Autodesk Fusion 360 part; units mm, degrees
sketch "Sketch1" plane through (0, 0, 0) normal (0, 0, 1) x (1, 0, 0)
  line L0 (-4.25, 7.25) -> (4.25, 7.25)
  line L1 (7.25, 4.25) -> (7.25, -4.25)
  line L2 (4.25, -7.25) -> (-4.25, -7.25)
  line L3 (-7.25, -4.25) -> (-7.25, 4.25)
  line L4 (-7.25, 7.25) -> (7.25, -7.25) construction
  line L5 (7.25, 7.25) -> (-7.25, -7.25) construction
  arc A0 (-4.25, 7.25) -> (-7.25, 4.25) centre (-4.25, 4.25) ccw
  arc A1 (-7.25, -4.25) -> (-4.25, -7.25) centre (-4.25, -4.25) ccw
  arc A2 (4.25, -7.25) -> (7.25, -4.25) centre (4.25, -4.25) ccw
  arc A3 (7.25, 4.25) -> (4.25, 7.25) centre (4.25, 4.25) ccw
  line L6 (10, 10) -> (-10, 10)
  line L7 (-15, 5) -> (-15, -5)
  line L8 (-10, -10) -> (10, -10)
  line L9 (15, -5) -> (15, 5)
  line L10 (15, 10) -> (-15, -10) construction
  line L11 (-15, 10) -> (15, -10) construction
  arc A4 (15, 5) -> (10, 10) centre (10, 5) ccw
  arc A5 (-10, 10) -> (-15, 5) centre (-10, 5) ccw
  arc A6 (-15, -5) -> (-10, -10) centre (-10, -5) ccw
  arc A7 (10, -10) -> (15, -5) centre (10, -5) ccw
  circle A8 centre (-12.5, 0) radius 1.6
  line L12 (0, 0) -> (0, 5.6259) construction
  circle A9 centre (12.5, 0) radius 1.6
  line L13 (-5.5, 2.65) -> (5.5, 2.65)
  line L14 (5.5, 2.65) -> (5.5, -2.65)
  line L15 (5.5, -2.65) -> (-5.5, -2.65)
  line L16 (-5.5, -2.65) -> (-5.5, 2.65)
  line L17 (-5.5, 2.65) -> (5.5, -2.65) construction
  line L18 (5.5, 2.65) -> (-5.5, -2.65) construction
  line L19 (-5.5, 1.4) -> (-5.5, -1.4)
  line L20 (-3, 4.4279) -> (-3, -3.4951) construction
  line L21 (-5.5, 1.4) -> (-3, 2.65)
  line L22 (-3, -2.65) -> (-5.5, -1.4)
  dimension "d1" = 14.5
  dimension "d2" = 14.5
  dimension "d3" = 3
  dimension "d4" = 30
  dimension "d5" = 20
  dimension "d6" = 5
  dimension "d7" = 3.2
  dimension "d8" = 11
  dimension "d9" = 5.3
  dimension "d10" = 2.8
  dimension "d11" = 2.5
  dimension "d12" = 1.4
  dimension "d17" = 12.5
extrude "Extrude1" add sketch "Sketch1" along normal blind 2.5 contours L0 L1 L2 L3 A0 A1 A2 A3 | L6 L7 L8 L9 A4 A5 A6 A7 | L13 L16 L21 | L15 L16 L22
extrude "Extrude2" add sketch "Sketch1" against normal blind 11 contours L0 L1 L2 L3 A0 A1 A2 A3 | L13 L16 L21 | L15 L16 L22
sketch "Sketch2" plane through (0, 0, -11) normal (0, 0, -1) x (-1, 0, 0)
  line L0 (5.5, 1.4) -> (5.5, -1.4)
  line L1 (5.5, -1.4) -> (3, -2.65)
  line L2 (3, -2.65) -> (-5.5, -2.65)
  line L3 (-5.5, -2.65) -> (-5.5, 2.65)
  line L4 (-5.5, 2.65) -> (3, 2.65)
  line L5 (3, 2.65) -> (5.5, 1.4)
  arc A0 (-7.25, -4.25) -> (-4.25, -7.25) centre (-4.25, -4.25) ccw
  line L6 (-4.25, -7.25) -> (4.25, -7.25)
  arc A1 (4.25, -7.25) -> (7.25, -4.25) centre (4.25, -4.25) ccw
  line L7 (7.25, -4.25) -> (7.25, 4.25)
  arc A2 (7.25, 4.25) -> (4.25, 7.25) centre (4.25, 4.25) ccw
  line L8 (4.25, 7.25) -> (-4.25, 7.25)
  arc A3 (-4.25, 7.25) -> (-7.25, 4.25) centre (-4.25, 4.25) ccw
  line L9 (-7.25, 4.25) -> (-7.25, -4.25)
  line L10 (5.9, -1.6472) -> (3.0944, -3.05)
  line L11 (3.0944, -3.05) -> (-5.9, -3.05)
  line L12 (-5.9, -3.05) -> (-5.9, 3.05)
  line L13 (-5.9, 3.05) -> (3.0944, 3.05)
  line L14 (3.0944, 3.05) -> (5.9, 1.6472)
  line L15 (5.9, 1.6472) -> (5.9, -1.6472)
  line L16 (5.7, 1.5236) -> (5.7, -1.5236)
  line L17 (5.7, -1.5236) -> (3.0472, -2.85)
  line L18 (3.0472, -2.85) -> (-5.7, -2.85)
  line L19 (-5.7, -2.85) -> (-5.7, 2.85)
  line L20 (-5.7, 2.85) -> (3.0472, 2.85)
  line L21 (3.0472, 2.85) -> (5.7, 1.5236)
  dimension "d18" = -0.4
  dimension "d21" = -0.2
extrude "Extrude3" cut sketch "Sketch2" against normal blind 2 contours L10 L11 L12 L13 L14 L15 | L16 L17 L18 L19 L20 L21
extrude "Extrude4" cut sketch "Sketch2" against normal through all contours L0 L1 L2 L3 L4 L5 | L16 L17 L18 L19 L20 L21
equation "d12 = d10 / 2"
Verification items for the finished model (mm, model axes). A direction names the side the tool comes from. Give positions to 0.01 mm unless a question says otherwise; leave off trailing zeros. Loops run counter-clockwise (first coordinate to the right, second up) from the corner with the lowest first, then second, coordinate; pieces in that order, holes last.
1. Thickness scan on line 1 (Y direction, x = 0.5, z = -4.75); line 2 (X direction, y = 2.25, z = -6.75); line 3 (Y direction, x = 0, z = 1.5). Record the ranges inside material, lowest first.
2. Go/stop test with flat-tipped pins: pin 1 Ø4 at (x, z) = (1, -4) entering from -Y; pin 2 Ø7 at (y, z) = (0, -4) entering from +X; pin 3 Ø8 at (x, z) = (9.5, -4.5) entering from +Y. Record where each tip stops, or that it passes through.
3. Section check D-D, the plane x = -12.5. Enter the section's corners in (y, z), then the cut area to 3 significant figures.
4. Set-up check for faces 1 (the flat face through (0, -7.25, -5)), 2 (the cylindrical face through (6.35, -6.39, -5.42)), 3 (the flat face through (1, -3.05, -10)), 4 (the cylindrical face through (6.39, 6.35, -5.42)): record each of +Z, -Z, +X, -X, +Y, -Y from which the full face is reachable in a straight line by a thin tool's end or side.
5. Section check A-A, the plane y = 0. Enter the section's corners in (x, z).
6. Mould release check, pull along Y, two halves, no side actions. Record for faces 5 (the flat face through (7.25, 0, -5)), 6 (the flat face through (1, -2.85, -3)), 7 (the flat face through (0, 10, 1)): released by +Y, released by -Y, zero draft, split by the parting line, or undercut.
7. Section check B-B, the plane z = 0.5. Enter the section's corners in (x, y).
8. Section check C-C, the plane z = -7.5. Enter the section's corners in (x, y).
Geometry says:
1. line 1: y = -7.25 to -2.85, 2.85 to 7.25
1. line 2: x = -7.25 to -4.25, 5.7 to 7.25
1. line 3: y = -10 to -2.85, 2.85 to 10
2. pin 1: stops at y = -7.25
2. pin 2: stops at x = 7.25
2. pin 3: stops at y = 6.98
3. outline: (-9.33, 0) - (-1.6, 0) - (-1.6, 2.5) - (-9.33, 2.5) - close; (1.6, 0) - (9.33, 0) - (9.33, 2.5) - (1.6, 2.5) - close
3. area: 38.7 mm2
4. face 1: -Z, +X, -X, -Y
4. face 2: -Z, +X, -Y
4. face 3: -Z
4. face 4: -Z, +X, +Y
5. outline: (-15, 0) - (-14.1, 0) - (-14.1, 2.5) - (-15, 2.5) - close; (-10.9, 0) - (-7.25, 0) - (-7.25, -11) - (-5.9, -11) - (-5.9, -9) - (-5.7, -9) - (-5.7, 2.5) - (-10.9, 2.5) - close; (5.7, -9) - (5.9, -9) - (5.9, -11) - (7.25, -11) - (7.25, 0) - (10.9, 0) - (10.9, 2.5) - (5.7, 2.5) - close; (14.1, 0) - (15, 0) - (15, 2.5) - (14.1, 2.5) - close
6. face 5: zero draft
6. face 6: undercut
6. face 7: released by +Y
7. outline: (-15, -5) arc R5 ccw to (-10, -10) - (10, -10) arc R5 ccw to (15, -5) - (15, 5) arc R5 ccw to (10, 10) - (-10, 10) arc R5 ccw to (-15, 5) - close; hole circle Ø3.2 at (-12.5, 0); hole (-5.7, -1.52) - (-3.05, -2.85) - (5.7, -2.85) - (5.7, 2.85) - (-3.05, 2.85) - (-5.7, 1.52) - close; hole circle Ø3.2 at (12.5, 0)
8. outline: (-7.25, -4.25) arc R3 ccw to (-4.25, -7.25) - (4.25, -7.25) arc R3 ccw to (7.25, -4.25) - (7.25, 4.25) arc R3 ccw to (4.25, 7.25) - (-4.25, 7.25) arc R3 ccw to (-7.25, 4.25) - close; hole (-5.7, -1.52) - (-3.05, -2.85) - (5.7, -2.85) - (5.7, 2.85) - (-3.05, 2.85) - (-5.7, 1.52) - close
